Input: part model. Units: mm. Frame: model coordinates. A direction names the side the tool comes from. Coordinates: 2 decimals unless noted, no trailing zeros. Order: outer loops, then holes, each group sorted by start corner. A loop starts at its lowest first (then second) coordinate and runs counter-clockwise, first axis right, second up. Notation, with made-up numbers: M -21.75,-10 L -6.75,-10 A22 cw -6.75,-1 Z; hole C -13,1 d8. An arc over 180 degrees is marked long. Answer in a Markdown table with one row per item.
from build123d import *

# Parameters (mm, degrees)
SKETCH1_R           = 32.5
BOSS_EXTRUDE1_DEPTH = 5
SKETCH3_R           = 34.5
BOSS_EXTRUDE3_DEPTH = 20
SKETCH2_R           = 1.25
SKETCH2_R_2         = 4
CUT_EXTRUDE1_DEPTH  = 11.5
SKETCH4_R           = 3.25
CUT_EXTRUDE2_DEPTH  = 21
SKETCH5_R           = 3.5
CUT_EXTRUDE3_DEPTH  = 21.5
CHAMFER1_SIZE       = 5


with BuildPart() as part:
    # Sketch1 → Boss-Extrude1 (new body)
    with BuildSketch(Plane(origin=(0, 0, 0), x_dir=(1, 0, 0), z_dir=(0, 1, 0))):
        with Locations(Location((0, 0, 0), (0, 0, 270))):
            Circle(SKETCH1_R)
    extrude(amount=BOSS_EXTRUDE1_DEPTH)

    # Sketch3 → Boss-Extrude3 (add)
    with BuildSketch(Plane(origin=(0, 5, 0), x_dir=(1, 0, 0), z_dir=(0, 1, 0))):
        with Locations(Location((0, 0, 0), (0, 0, 270))):
            Circle(SKETCH3_R)
    extrude(amount=BOSS_EXTRUDE3_DEPTH)

    # Sketch2 → Cut-Extrude1 (cut)
    with BuildSketch(Plane(origin=(0, 0, 0), x_dir=(1, 0, 0), z_dir=(0, 1, 0))):
        with Locations(Location((-5, 8.660254038, 0), (0, 0, 270))):
            Circle(SKETCH2_R)
        with Locations(Location((5, 8.660254038, 0), (0, 0, 270))):
            Circle(SKETCH2_R)
        with Locations(Location((10, 0, 0), (0, 0, 270))):
            Circle(SKETCH2_R)
        with Locations(Location((5, -8.660254038, 0), (0, 0, 270))):
            Circle(SKETCH2_R)
        with Locations(Location((-5, -8.660254038, 0), (0, 0, 270))):
            Circle(SKETCH2_R)
        with Locations(Location((-10, 0, 0), (0, 0, 270))):
            Circle(SKETCH2_R)
        with Locations(Location((0, 0, 0), (0, 0, 270))):
            Circle(SKETCH2_R_2)
    extrude(amount=CUT_EXTRUDE1_DEPTH, mode=Mode.SUBTRACT)

    # Sketch4 → Cut-Extrude2 (cut)
    with BuildSketch(Plane(origin=(0, 25, 0), x_dir=(1, 0, 0), z_dir=(0, 1, 0))):
        with Locations(Location((10, 0, 0), (0, 0, 270))):
            Circle(SKETCH4_R)
        with Locations(Location((5, 8.660254038, 0), (0, 0, 270))):
            Circle(SKETCH4_R)
        with Locations(Location((5, -8.660254038, 0), (0, 0, 270))):
            Circle(SKETCH4_R)
        with Locations(Location((-5, -8.660254038, 0), (0, 0, 270))):
            Circle(SKETCH4_R)
        with Locations(Location((-10, 0, 0), (0, 0, 270))):
            Circle(SKETCH4_R)
        with Locations(Location((-5, 8.660254038, 0), (0, 0, 270))):
            Circle(SKETCH4_R)
    extrude(amount=-CUT_EXTRUDE2_DEPTH, mode=Mode.SUBTRACT)

    # Sketch5 → Cut-Extrude3 (cut)
    with BuildSketch(Plane(origin=(0, 25, 0), x_dir=(1, 0, 0), z_dir=(0, 1, 0))):
        with Locations(Location((0, 20, 0), (0, 0, 270))):
            Circle(SKETCH5_R)
        with Locations(Location((20, 0, 0), (0, 0, 270))):
            Circle(SKETCH5_R)
        with Locations(Location((0, -20, 0), (0, 0, 270))):
            Circle(SKETCH5_R)
        with Locations(Location((-20, 0, 0), (0, 0, 270))):
            Circle(SKETCH5_R)
    extrude(amount=-CUT_EXTRUDE3_DEPTH, mode=Mode.SUBTRACT)

    # Chamfer1
    chamfer1_edges = [part.edges().sort_by_distance(p)[0] for p in [
        (0, 25, -34.5),
    ]]
    chamfer(chamfer1_edges, length=CHAMFER1_SIZE)


solid = part.part
1) Cut plane A-A, the plane y = 14. State how many separate pieces and enclosed holes the cut face has, and give its area (3 significant figures).
Resolved:
| item | result |
|---|---|
| separate pieces | 1 |
| enclosed holes | 10 |
| area | 3,390 mm2 |
2) Material intervals for probe 1 along X at (y, z) = (2.7, 0); probe 2 along X at (y, z) = (12.75, 0); probe 3 along Z at (x, y) = (6, 1.5), sorted ascending.
Resolved:
| item | result |
|---|---|
| probe 1 | x = -32.5 to -11.25, -8.75 to -4, 4 to 8.75, 11.25 to 32.5 |
| probe 2 | x = -34.5 to -23.5, -16.5 to -13.25, -6.75 to 6.75, 13.25 to 16.5, 23.5 to 34.5 |
| probe 3 | z = -31.94 to -9.41, -7.91 to 7.91, 9.41 to 31.94 |
3) Reachability of faces 5 (the face through (-13, 5, 31)), 6 (the face through (1.05, 14.4, -16.66)), 7 (the face through (4.521, 1.972, -7.506)) from +Z, -Z, +X, -X, +Y, -Y: full face, straight path, thin tool, end or side. Return the list, or none.
Resolved:
| item | result |
|---|---|
| face 5 | -Y |
| face 6 | +Y |
| face 7 | +Y, -Y |
4) Mould query, pull axis X, two halves, no side actions, for faces 1 (the face through (-6.778, 14.647, -0.423)), 2 (the face through (0, 25, 0)), 3 (the face through (7.74, 14.65, 10.41)), 4 (the face through (1.517, 12.395, -34.467)). Classes: +X half, -X half, draft (parallel to the pull), parting line (faces both ways), or undercut.
Resolved:
| item | result |
|---|---|
| face 1 | undercut |
| face 2 | draft |
| face 3 | undercut |
| face 4 | parting line |
5) Contact query for flat-ended pins moving along their axis: pin 1 (3 mm diameter, centred on x = 5, z = 8.66, fed in from +Y); pin 2 (8 mm diameter, centred on x = 14, y = 19, fed in from -Z); pin 3 (1.5 mm diameter, centred on x = -5, z = -8.66, fed in from +Y); pin 4 (6 mm diameter, centred on x = -27, z = 25.5, fed in from +Y). Output: stop coordinate, or through.
Resolved:
| item | result |
|---|---|
| pin 1 | stops at y = 4 |
| pin 2 | stops at z = -33.02 |
| pin 3 | passes through |
| pin 4 | stops at y = 20.36 |
6) Cut plane C-C, the plane x = 0. Output: boundary loops of the cut face in (y, z).
Resolved:
| item | result |
|---|---|
| outline | M 0,-32.5 L 5,-32.5 L 5,-34.5 L 20,-34.5 L 25,-29.5 L 25,-23.5 L 3.5,-23.5 L 3.5,-16.5 L 25,-16.5 L 25,16.5 L 3.5,16.5 L 3.5,23.5 L 25,23.5 L 25,29.5 L 20,34.5 L 5,34.5 L 5,32.5 L 0,32.5 L 0,4 L 11.5,4 L 11.5,-4 L 0,-4 Z |
